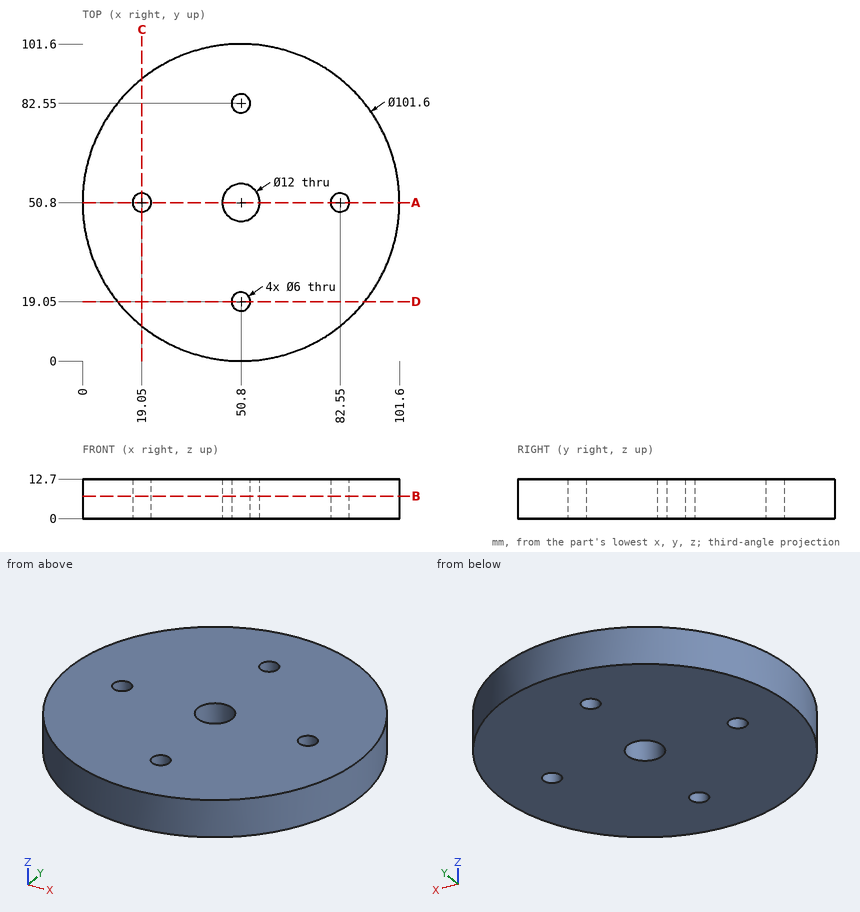
Verification items for this drawing (mm, ordinates from the low corner). Give positions to 0.01 mm unless a question says otherwise; leave off trailing zeros. Write each loop counter-clockwise with the first axis right and the second up, starting at its lowest first coordinate (ties: lowest second). Pieces come first, ordered by that corner, then holes. Notation, with made-up numbers: M 48.5,-16 L 103.5,-16 A31 ccw 103.5,9 Z; hole C 22.25,-16 d7. An arc over 180 degrees is marked long. Use one line per item in the form item = value.
(1) Material ranges on line 1 along Y through (x, z) = (53, 11); line 2 along Y through (x, z) = (50.8, 6.25); line 3 along X through (y, z) = (52, 5.75), recorded low to high.
Answer block:
line_1 = 0.05 to 17.01, 21.09 to 45.22, 56.38 to 80.51, 84.59 to 101.55
line_2 = 0 to 16.05, 22.05 to 44.8, 56.8 to 79.55, 85.55 to 101.6
line_3 = 0.01 to 16.3, 21.8 to 44.92, 56.68 to 79.8, 85.3 to 101.59
(2) Section check B-B on z = 7.25. Record the boundary of the cut face in (x, y), plus the area to 3 significant figures.
Answer block:
outline = C 50.8,50.8 d101.6; hole C 19.05,50.8 d6; hole C 50.8,50.8 d12; hole C 50.8,19.05 d6; hole C 50.8,82.55 d6; hole C 82.55,50.8 d6
area = 7,880 mm2
(3) Section check A-A on y = 50.8. Record the boundary of the cut face in (x, z), plus the area to 3 significant figures.
Answer block:
outline = M 0,0 L 16.05,0 L 16.05,12.7 L 0,12.7 Z; M 22.05,0 L 44.8,0 L 44.8,12.7 L 22.05,12.7 Z; M 56.8,0 L 79.55,0 L 79.55,12.7 L 56.8,12.7 Z; M 85.55,0 L 101.6,0 L 101.6,12.7 L 85.55,12.7 Z
area = 986 mm2
(4) Section check C-C on x = 19.05. Record the boundary of the cut face in (y, z), plus the area to 3 significant figures.
Answer block:
outline = M 11.14,0 L 47.8,0 L 47.8,12.7 L 11.14,12.7 Z; M 53.8,0 L 90.46,0 L 90.46,12.7 L 53.8,12.7 Z
area = 931 mm2
(5) Depth check by flat-ended pin: P1, Ø3, axis at x = 86, z = 4.5, coming from the -Y side; P2, Ø15.5, axis at x = 50.8, y = 50.8, coming from the +Z side; P3, Ø4, axis at x = 29, z = 3, coming from the +Y side. Enter the tip coordinate at first touch or a pass-through.
Answer block:
P1 = 12.79
P2 = 12.7
P3 = 97.58
